```python
from build123d import *

# Parameters (mm, degrees)
F0_W        = 100
F0_H        = 100
F0_R        = 5
F0_R_2      = 5.515434
F0_R_3      = 32
F1_DEPTH    = 2.5
F1_FACE_W   = 100
F1_FACE_H   = 100
F1_FACE_R   = 5
F1_FACE_R_2 = 5.515434
F2_DEPTH    = 3.5
F3_R        = 30
F4_DEPTH    = 25


with BuildPart() as f1:
    # F0 (on Front) → F1 (new body)
    with BuildSketch(Plane.XZ):
        Rectangle(F0_W, F0_H)
        with Locations((-40.200002, -41.250005)):
            Circle(F0_R, mode=Mode.SUBTRACT)
        with Locations((40.5, -41.250005)):
            Circle(F0_R, mode=Mode.SUBTRACT)
        with Locations((-40.5, 40.350001)):
            Circle(F0_R_2, mode=Mode.SUBTRACT)
        Circle(F0_R_3, mode=Mode.SUBTRACT)
        with Locations((40.799998, 40.950008)):
            Circle(F0_R, mode=Mode.SUBTRACT)
        Circle(F0_R_3)
    extrude(amount=F1_DEPTH)

    # F0 (on Front) + F1_face (on face) → F2 (join)
    with BuildSketch(Plane.XZ):
        Circle(F0_R_3)
    with BuildSketch(Plane(origin=(0.06645, -2.5, -0.061312), x_dir=(1, 0, 0), z_dir=(0, -1, 0))):
        with Locations((-0.06645, 0.061312)):
            Rectangle(F1_FACE_W, F1_FACE_H)
        with Locations((-40.266452, -41.188694)):
            Circle(F1_FACE_R, mode=Mode.SUBTRACT)
        with Locations((40.43355, -41.188694)):
            Circle(F1_FACE_R, mode=Mode.SUBTRACT)
        with Locations((-40.56645, 40.411313)):
            Circle(F1_FACE_R_2, mode=Mode.SUBTRACT)
        with Locations((40.733548, 41.011319)):
            Circle(F1_FACE_R, mode=Mode.SUBTRACT)
    extrude(amount=-F2_DEPTH)

    # F3 (on face) → F4 (cut)
    with BuildSketch(Plane(origin=(0, 3.5, 0), x_dir=(-1, 0, 0), z_dir=(0, 1, 0))):
        Circle(F3_R)
    extrude(amount=-F4_DEPTH, mode=Mode.SUBTRACT)


solid = f1.part
```
Geometry: final body of the model. Coordinates: model frame, mm. A direction names the side the tool comes from. Round coordinates to 2 decimals unless told otherwise and drop trailing zeros. Order: outer loops, then holes, each group sorted by start corner. A loop starts at its lowest first (then second) coordinate and runs counter-clockwise, first axis right, second up. Notation, with made-up numbers: (51, -29.75) -> (86, -29.75) arc R23 ccw to (86, -13.75) -> close; hole circle Ø3 at (48, 3). An arc over 180 degrees is marked (long way). Use one line per item in the form item = value.
(1) Section B-B on z = 0. Return loops of the section in (x, y), and give its area (3 significant figures).
Results list:
outline = (-50, -2.5) -> (-30, -2.5) -> (-30, 3.5) -> (-32, 3.5) -> (-32, 1) -> (-50, 1) -> close; (30, -2.5) -> (50, -2.5) -> (50, 1) -> (32, 1) -> (32, 3.5) -> (30, 3.5) -> close
area = 150 mm^2
(2) Ray query, probe 1 along Z at (x, y) = (40.5, -1.7); probe 2 along Z at (x, y) = (-40.5, -1.55); probe 3 along Y at (x, z) = (7, -44.5). Return the intervals inside material, ascending. Write a range as [from, to].
Results list:
probe_1 = [-50, -46.25], [-36.25, 35.96], [45.94, 50]
probe_2 = [-50, -46.24], [-36.26, 34.83], [45.87, 50]
probe_3 = [-2.5, 1]
(3) Section A-A on x = 0. Return loops of the section in (y, z).
Results list:
outline = (-2.5, -50) -> (1, -50) -> (1, -32) -> (3.5, -32) -> (3.5, -30) -> (-2.5, -30) -> close; (-2.5, 30) -> (3.5, 30) -> (3.5, 32) -> (1, 32) -> (1, 50) -> (-2.5, 50) -> close
(4) Draft query along X for faces 3 (the face through (-23, 1, 23)), 4 (the face through (-37.95, -0.77, 35.46)), 5 (the face through (50, -1, -1)), 6 (the face through (-50, -1, -1)). Return one class per face: pulls with the +X half, pulls with the -X half, needs draft (parallel to the pull), parting line crosses it, or undercut.
Results list:
face_3 = needs draft
face_4 = undercut
face_5 = pulls with the +X half
face_6 = pulls with the -X half
(5) Access query for faces 1 (the face through (-1, -1, -50)), 2 (the face through (-6.94, 2.23, -31.24)). Directions: +Z, -Z, +X, -X, +Y, -Y. A direction counts if a zero-diameter tool reaches every point of the face in a straight line with its end or side. Return the directions, or none.
Results list:
face_1 = -Z, +X, -X, +Y, -Y
face_2 = +Y
